Autodesk Inventor part; units mm, degrees
ref_plane "Work Plane3" through (-28.575, 0, 0) normal (0, 0, -1) x (-1, 0, 0)
ref_plane "YZ Plane" through (0, 0, 0) normal (1, 0, 0) x (0, 1, 0)
ref_plane "XZ Plane" through (0, 0, 0) normal (0, 1, 0) x (-1, 0, 0)
sketch "Sketch1" plane through (0, 0, 0) normal (1, 0, 0) x (0, 1, 0)
  circle A0 centre (0, 0) radius 14.2875
  circle A1 centre (0, 0) radius 12.7
  dimension "d0" = 28.575
  dimension "d1" = 25.4
extrude "Extrusion1" add sketch "Sketch1" along normal blind 152.4
sketch "Sketch2" plane through (0, 0, 0) normal (-1, 0, 0) x (0, 0, 1)
  circle A0 centre (0, 0) radius 14.2875
extrude "Extrusion2" add sketch "Sketch2" along normal blind 3.175
sketch "Sketch3" plane through (-3.175, 0, 0) normal (-1, 0, 0) x (0, 0, 1)
  circle A0 centre (0, 0) radius 6.35
  dimension "d6" = 12.7
extrude "Extrusion3" add sketch "Sketch3" along normal blind 25.4
sketch "Sketch4" plane through (-28.575, 0, 0) normal (-1, 0, 0) x (0, 0, 1)
  circle A0 centre (0, 0) radius 6.35
  circle A1 centre (0, 0) radius 6.35
  point P0 (6.35, 0)
  point P1 (-6.35, 0)
ref_plane "Work Plane3" through (-28.575, 0, 0) normal (0, 0, -1) x (-1, 0, 0)
ref_plane "Work Plane1" through (-28.575, 0, 6.35) normal (0, 0, 1) x (1, 0, 0)
ref_plane "Work Plane2" through (-28.575, 0, -6.35) normal (0, 0, -1) x (-1, 0, 0)
sketch "Sketch5" plane through (-28.575, 0, 6.35) normal (0, 0, 1) x (1, 0, 0)
  circle A0 centre (6.35, 0) radius 3.175
  line L0 (0, 6.35) -> (0, -6.35)
  point P0 (28.575, 0)
  dimension "d9" = 6.35
  dimension "d10" = 6.35
extrude "Extrusion4" cut sketch "Sketch5" against normal blind 25.4
properties part number "Intake Basic Piston - Outer"
Could you check a few things on this model? Use its own coordinates, in mm. A direction names the side the tool comes from. Coordinates: 2 decimals unless noted, no trailing zeros. Write each loop counter-clockwise with the first axis right and the second up, starting at its lowest first coordinate (ties: lowest second). Pieces come first, ordered by that corner, then holes. Notation, with made-up numbers: (37.25, 68) -> (80.25, 68) arc R8 ccw to (80.25, 79) -> close; hole circle Ø11 at (20.5, -5). An arc over 180 degrees is marked (long way). Return JSON: item names as keys, results as strings.
(1) We'd pull the mould along Y, two halves only. Please class faces 1 (the cylindrical face through (75.13, -2.75, 12.4)), 2 (the flat face through (-28.575, 0, 0)), 3 (the cylindrical face through (-20.52, 2.68, 0.09)), 4 (the cylindrical face through (73.523, -8.826, 11.236)): +Y half, -Y half, draft (parallel to the pull), parting line (faces both ways), or undercut.
Numbers:
{"face 1": "undercut", "face 2": "draft", "face 3": "undercut", "face 4": "parting line"}
(2) Imagine slicing it at C-C, the plane z = -11. Please give me the cut outline in (x, y) (3 decimals), then the cut area to 3 significant figures.
Numbers:
{"outline": "(-3.175, -9.118) -> (152.4, -9.118) -> (152.4, -6.347) -> (0, -6.347) -> (0, 6.347) -> (152.4, 6.347) -> (152.4, 9.118) -> (-3.175, 9.118) -> close", "area": "902 mm2"}
(3) Which directions (+Z, -Z, +X, -X, +Y, -Y) give clear straight access to the entire face, cutting with the end or side of a thin tool? Please do faces 5 (the flat face through (0, 0, 0)), 6 (the flat face through (152.4, -13, -1)), 7 (the flat face through (-3.175, -3, 6)).
Numbers:
{"face 5": "+X", "face 6": "+Z, -Z, +X, +Y, -Y", "face 7": "-X"}
(4) I need wall thicknesses on L1, parallel to X at y = 0, z = 2.25 (3 decimals); L2, parallel to Z at x = 122, y = 0; L3, parallel to X at y = 8, z = 6 (3 decimals). Which ranges of each line are inside material? Lowest first, please.
Numbers:
{"L1": "x = -28.575 to -25.4, -19.05 to 0", "L2": "z = -14.29 to -12.7, 12.7 to 14.29", "L3": "x = -3.175 to 0"}
(5) Imagine slicing it at B-B, the plane x = 54. Please give me the cut outline in (y, z) (1 decimal).
Numbers:
{"outline": "circle Ø28.6 at (0, 0); hole circle Ø25.4 at (0, 0)"}
(6) Imagine slicing it at A-A, the plane y = -10. Please give me the cut outline in (x, z) (3 decimals), then the cut area to 3 significant figures.
Numbers:
{"outline": "(-3.175, -10.205) -> (152.4, -10.205) -> (152.4, -7.829) -> (0, -7.829) -> (0, 7.829) -> (152.4, 7.829) -> (152.4, 10.205) -> (-3.175, 10.205) -> close", "area": "789 mm2"}
(7) I'm going to push flat-ended pins straight in: pin 1 (1 mm diameter, centred on x = 101, y = 5, fed in from +Z); pin 2 (1.5 mm diameter, centred on x = 39.5, z = -8, fed in from +Y); pin 3 (7.5 mm diameter, centred on x = -22.225, y = 0, fed in from +Z). Where does each tip first touch, or does it pass through?
Numbers:
{"pin 1": "stops at z = 13.56", "pin 2": "stops at y = 12.31", "pin 3": "stops at z = 6.35"}
